```python
from build123d import *

# Parameters (mm, degrees)
BOSS_EXTRUDE1_DEPTH      = 31.8
CUT_EXTRUDE1_REACH       = 35.336
CUT_EXTRUDE1_END_RADIUS  = 57.3
SKETCH2_W                = 29.4
SKETCH2_H                = 13.3
BOSS_EXTRUDE2_REACH      = 35.336
BOSS_EXTRUDE2_END_RADIUS = 57.3
SKETCH3_R                = 3.25
SKETCH3_R_2              = 2.4
SKETCH4_R                = 3.25
SKETCH4_R_2              = 2.4
CUT_EXTRUDE2_DEPTH       = 0.2
LPATTERN1_COUNT          = 2
LPATTERN1_PITCH          = 8
LPATTERN2_COUNT          = 2
LPATTERN2_PITCH          = 8
SKETCH5_W                = 29.4
SKETCH5_H                = 2.5
CUT_EXTRUDE3_DEPTH       = 0.3


with BuildPart() as part:
    # Sketch1 → Boss-Extrude1 (new body)
    with BuildSketch(Plane(origin=(0, 0, 0), x_dir=(0, 0, -1), z_dir=(1, 0, 0))):
        with BuildLine():
            Line((-7.85, 0), (7.85, 0))
            Line((7.85, 0), (7.85, 6.2))
            ThreePointArc((7.85, 6.2), (-0.147838397, 4.652634009), (-7.85, 2))
            Line((-7.85, 2), (-7.85, 0))
        make_face()
    extrude(amount=-BOSS_EXTRUDE1_DEPTH)

    # Cut-Extrude1: up to this cylinder (the profile starts inside it)
    cut_extrude1_end = Plane(origin=(-15.9, -51.377128325, -14.841015221), z_dir=(1, 0, 0)) * Cylinder(CUT_EXTRUDE1_END_RADIUS, 186.272, mode=Mode.PRIVATE)
    # Sketch2 → Cut-Extrude1 (cut, up to the surface)
    with BuildSketch(Plane.XZ, mode=Mode.PRIVATE) as cut_extrude1_sk1:
        with Locations((-15.9, 0)):
            Rectangle(SKETCH2_W, SKETCH2_H)
    cut_extrude1_tool1 = extrude(cut_extrude1_sk1.sketch, amount=-CUT_EXTRUDE1_REACH, mode=Mode.PRIVATE) & cut_extrude1_end
    add(cut_extrude1_tool1.solids().sort_by_distance((-15.9, 0, 0))[0], mode=Mode.SUBTRACT)

    # Boss-Extrude2: up to this cylinder (the profile starts inside it)
    boss_extrude2_end = Plane(origin=(-15.9, -51.377128325, -14.841015221), z_dir=(1, 0, 0)) * Cylinder(BOSS_EXTRUDE2_END_RADIUS, 186.272, mode=Mode.PRIVATE)
    # Sketch3 → Boss-Extrude2 (add, up to the surface)
    with BuildSketch(Plane.XZ, mode=Mode.PRIVATE) as boss_extrude2_sk1:
        with Locations(Location((-15.9, 0, 0), (0, 0, 270))):
            Circle(SKETCH3_R)
        with Locations(Location((-15.9, 0, 0), (0, 0, 270))):
            Circle(SKETCH3_R_2, mode=Mode.SUBTRACT)
    boss_extrude2_tool1 = extrude(boss_extrude2_sk1.sketch, amount=-BOSS_EXTRUDE2_REACH, mode=Mode.PRIVATE) & boss_extrude2_end
    boss_extrude2 = boss_extrude2_tool1.solids().sort_by_distance((-15.9, 0, 3.158076))[0]
    add(boss_extrude2)

    # Sketch4 → Cut-Extrude2 (cut)
    with BuildSketch(Plane.XZ):
        with Locations(Location((-15.9, 0, 0), (0, 0, 270))):
            Circle(SKETCH4_R)
        with Locations(Location((-15.9, 0, 0), (0, 0, 270))):
            Circle(SKETCH4_R_2, mode=Mode.SUBTRACT)
    cut_extrude2 = extrude(amount=-CUT_EXTRUDE2_DEPTH, mode=Mode.SUBTRACT)

    # LPattern1: Boss-Extrude2, Cut-Extrude2 ×2
    with Locations(*[(i * LPATTERN1_PITCH, 0, 0) for i in range(1, LPATTERN1_COUNT)]):
        add(boss_extrude2)
        add(cut_extrude2, mode=Mode.SUBTRACT)

    # LPattern2: Boss-Extrude2, Cut-Extrude2 ×2
    with Locations(*[(-i * LPATTERN2_PITCH, 0, 0) for i in range(1, LPATTERN2_COUNT)]):
        add(boss_extrude2)
        add(cut_extrude2, mode=Mode.SUBTRACT)

    # Sketch5 → Cut-Extrude3 (cut)
    with BuildSketch(Plane(origin=(0, 2, 0), x_dir=(-1, 0, 0), z_dir=(0, -1, 0))):
        with Locations((15.9, -5.4)):
            Rectangle(SKETCH5_W, SKETCH5_H)
    extrude(amount=-CUT_EXTRUDE3_DEPTH, mode=Mode.SUBTRACT)


solid = part.part
```
The model under review builds one solid part; all positions refer to its coordinate system, in mm. A direction names the side the tool comes from. Give positions to 0.01 mm unless a question says otherwise; leave off trailing zeros. Loops run counter-clockwise (first coordinate to the right, second up) from the corner with the lowest first, then second, coordinate; pieces in that order, holes last. Notation, with made-up numbers: (23.25, 49.25) - (49.25, 49.25) arc R12 ccw to (49.25, 64.25) - close; hole circle Ø4 at (8.25, -31.5). An arc over 180 degrees is marked (long way). Answer as a JSON object with one key per item and string values.
Q1. Insertion check: pin 1 (7 mm diameter, centred on x = -24, z = 0.5, fed in from -Y); pin 2 (4 mm diameter, centred on x = -15.9, z = 0, fed in from -Y); pin 3 (3 mm diameter, centred on x = -20, z = -5, fed in from -Y). Each pin has a flat end and moves straight along its axis. Give the tip position at first contact, or say it passes through.
Worked out:
{"pin 1": "stops at y = 0.2", "pin 2": "stops at y = 3.39", "pin 3": "stops at y = 4.79"}
Q2. Add section A-A on x = -15.5. State the section outline as (y, z) points, plus the area to 3 significant figures.
Worked out:
{"outline": "(0, -7.85) - (6.2, -7.85) arc R58 ccw to (2, 7.85) - (0, 7.85) - (0, 6.65) - (1.74, 6.65) arc R57.3 cw to (2, 6) - (2, 6.65) - (2.3, 6.65) - (2.3, 5.21) arc R57.3 cw to (3, 3.23) - (0.2, 3.23) - (0.2, 2.37) - (3.28, 2.37) arc R57.3 cw to (4.55, -2.37) - (0.2, -2.37) - (0.2, -3.23) - (4.73, -3.23) arc R57.3 cw to (5.33, -6.65) - (0, -6.65) - close", "area": "25.7 mm^2"}
Q3. Add section B-B on z = 5.5. State the section outline as (x, y) points, plus the area to 3 significant figures.
Worked out:
{"outline": "(-31.8, 0) - (-30.6, 0) - (-30.6, 2.3) - (-1.2, 2.3) - (-1.2, 0) - (0, 0) - (0, 2.94) - (-31.8, 2.94) - close", "area": "25.8 mm^2"}
Q4. For faces 1 (the cylindrical face through (-22.92, 1.93, -3.1)), 2 (the flat face through (-16, 2.3, 6)), list the 3-axis set-ups (+Z, -Z, +X, -X, +Y, -Y) from which the entire face can be reached by the end or side of a thin tool; tool diameter is ignored.
Worked out:
{"face 1": "-Y", "face 2": "none"}
Q5. To check wall thickness, follow line 1 along Z through (x, y) = (-15.9, 1.7); line 2 along X through (y, z) = (2.5, -2.5); line 3 along Z through (x, y) = (-16, 2.25). State the ranges of each line that lie inside material, in increasing order.
Worked out:
{"line 1": "z = -7.85 to -6.65, -3.25 to -2.4, 2.4 to 3.25, 6.65 to 7.85", "line 2": "x = -31.8 to -30.6, -25.98 to -21.82, -17.98 to -13.82, -9.98 to -5.82, -1.2 to 0", "line 3": "z = -7.85 to -6.65, -3.25 to -2.4, 2.4 to 3.25, 6.65 to 7.25"}
Q6. Mouldability with a two-part tool opening along Z and no side actions: class faces 3 (the flat face through (-16, 3, -7.85)), 4 (the cylindrical face through (-15.68, 4.68, 0.04)), 5 (the flat face through (-16, 1, 6.65)), 6 (the flat face through (-15, 0, 7)) as +Z half, -Z half, draft (parallel to the pull), parting line (faces both ways), or undercut.
Worked out:
{"face 3": "-Z half", "face 4": "+Z half", "face 5": "undercut", "face 6": "draft"}
Q7. Add section C-C on x = -21. State the section outline as (y, z) points.
Worked out:
{"outline": "(0, -7.85) - (6.2, -7.85) arc R58 ccw to (2, 7.85) - (0, 7.85) - (0, 6.65) - (1.74, 6.65) arc R57.3 cw to (2, 6) - (2, 6.65) - (2.3, 6.65) - (2.3, 5.21) arc R57.3 cw to (3.55, 1.47) - (0.2, 1.47) - (0.2, -1.47) - (4.34, -1.47) arc R57.3 cw to (5.33, -6.65) - (0, -6.65) - close"}
